Solid Edge part; units mm, degrees
sketch "Sketch1" plane through (0, 0, 0) normal (0, 0, 1) x (1, 0, 0)
  arc A0 (-1.8, 0) -> (-1.0449, 2.0645) centre (1.4, 0) cw
  arc A1 (-1.0449, 2.0645) -> (-0.9685, 2.1) centre (-0.9685, 2) cw
  line L0 (-0.9685, 2.1) -> (0, 2.1)
  line L1 (0, 2.1) -> (0, 1.2)
  arc A2 (0, 1.2) -> (0.1, 1.1) centre (0.1, 1.2) ccw
  line L2 (0.1, 1.1) -> (7.5, 1.1)
  line L3 (7.5, 1.1) -> (9.5, 0)
  line L4 (9.5, 0) -> (-1.8, 0)
revolve "RevolvedProtrusion1" add sketch "Sketch1" angle 360 about axis through (12.5, 0, 0) along (-1, 0, 0)
cosmetic_thread "Thread1"
sketch "Sketch2" plane through (0, 0, 0) normal (0, 0, 1) x (1, 0, 0)
  line L0 (-1.8, -1) -> (-1.2, -1)
  line L1 (-1.2, -1) -> (-0.6, -0.4)
  line L2 (-0.6, -0.4) -> (-0.6, 0.4)
  line L3 (-0.6, 0.4) -> (-1.2, 1)
  line L4 (-1.2, 1) -> (-1.8, 1)
  line L5 (-1.8, 1) -> (-1.8, -1)
extrude "ExtrudedCutout_1" cut sketch "Sketch2" against normal blind 0.25 and the other way blind 0.25
sketch "Sketch3" plane through (0, 0, 0) normal (0, -1, 0) x (1, 0, 0)
  line L0 (-1.9, 1) -> (-1.21, 1)
  line L1 (-1.21, 1) -> (-0.61, 0.4)
  line L2 (-0.61, 0.4) -> (-0.61, -0.4)
  line L3 (-0.61, -0.4) -> (-1.21, -1)
  line L4 (-1.21, -1) -> (-1.9, -1)
  line L5 (-1.9, -1) -> (-1.9, 1)
extrude "ExtrudedCutout_2" cut sketch "Sketch3" against normal blind 0.25 and the other way blind 0.25
sketch "Sketch4" plane through (-0.8, 0, 0) normal (1, 0, 0) x (0, 1, 0)
  line L0 (-0.7071, 0.7071) -> (-0.1138, 0)
  line L1 (-0.1138, 0) -> (-0.7071, -0.7071)
  line L2 (-0.7071, -0.7071) -> (0, -0.1138)
  line L3 (0, -0.1138) -> (0.7071, -0.7071)
  line L4 (0.7071, -0.7071) -> (0.1138, 0)
  line L5 (0.1138, 0) -> (0.7071, 0.7071)
  line L6 (0.7071, 0.7071) -> (0, 0.1138)
  line L7 (0, 0.1138) -> (-0.7071, 0.7071)
extrude "ExtrudedCutout_3" cut sketch "Sketch4" against normal blind 1.8
properties part number "bene_inox_412405-2,2X9,5"
Build history of the part. All positions in model axes, mm. A direction names the side the tool comes from. Round coordinates to 2 decimals unless told otherwise and drop trailing zeros. Loops run counter-clockwise (first coordinate to the right, second up) from the corner with the lowest first, then second, coordinate; pieces in that order, holes last.
Item 1: Two-plate mould, pull along Y, no slides. Class faces 3 (the face through (0, 1, 1)), 4 (the face through (8.708, -0.435, -0.019)): released by +Y, released by -Y, zero draft, split by the parting line, or undercut.
Item 2: Drill centre lines: line 1 along Y through (x, z) = (8.5, -0.2); line 2 along X through (y, z) = (0.1, -1.55); line 3 along Z through (x, y) = (6.25, -0.9). Where is each one in solid material? Low to high.
Item 3: Which spindle directions (+Z, -Z, +X, -X, +Y, -Y) get a long thin tool onto all of the face, cutting with end or side? Do faces 1 (the face through (3.85, 1.05, 0.33)), 2 (the face through (-0.477, 2.003, 0.631)). Say none if no direction does.
Item 4: Saw through at A-A (x = 0.5). List the corners of the cut face in (y, z), then the cut area to 3 significant figures.
Item 5: Pin check, flat tips, straight feed: P1, Ø2, axis at y = -0.5, z = 0, coming from the -X side; P2, Ø2, axis at x = 8, y = 1.5, coming from the -Z side; P3, Ø0.6, axis at x = -1.5, y = 0, coming from the -Z side; P4, Ø1, axis at x = 6, z = 0.5, coming from the -Y side. Stop position of each tip, or through.
Worked answers:
1. face 3: zero draft
1. face 4: split by the parting line
2. line 1: y = -0.51 to 0.51
2. line 2: x = -1.4 to 0
2. line 3: z = -0.63 to 0.63
3. face 1: +X
3. face 2: +X, -X
4. outline: circle Ø2.2 at (0, 0)
4. area: 3.80 mm2
5. P1: stops at x = -1.77
5. P2: stops at z = -0.9
5. P3: stops at z = -1.87
5. P4: stops at y = -1.1
